Read the model definition and answer for the solid it produces. Units are mm, in the model's axes. Face numbers are marked on the shaded views. A direction names the side the tool comes from. Give positions to 0.01 mm unless a question says otherwise; leave off trailing zeros. Loops run counter-clockwise (first coordinate to the right, second up) from the corner with the lowest first, then second, coordinate; pieces in that order, holes last. Notation, with made-up numbers: (66, 65.5) - (112, 65.5) arc R15 ccw to (112, 84.5) - close; hole circle Ø2 at (56.25, 1.5). An arc over 180 degrees is marked (long way). Use a Markdown table: item, result. Add a question column.
Item 1: For a pull along Y with two mould halves and no side action, classify the marked faces 3, 4, 5 and 6 as +Y half, -Y half, draft (parallel to the pull), parting line (faces both ways), or undercut.
Item 2: Consider probe 1 along X at (y, z) = (19.5, 25.5); probe 2 along Y at (x, z) = (5.5, 19.75); probe 3 along X at (y, z) = (10, 24). Determine where each line is inside the solid, lowest interval first. Write a range as [from, to].
Item 3: A cutting plane is placed at C-C (x = -20). Determine the outline of the cut face in (y, z), plus the area to 3 significant figures.
Item 4: Which of the six approach directions +Z, -Z, +X, -X, +Y, -Y give full straight-line access (tool end or side, diameter ignored) to the marked faces 1 and 2?
Item 5: A cutting plane is placed at B-B (z = 25). Determine the outline of the cut face in (x, y).
Item 6: A cutting plane is placed at D-D (z = 19.75). Determine the outline of the cut face in (x, y).
Item 7: Each of these flat-tipped pins is pushed along its axis until it touches: P1, Ø5, axis at x = -20.44, y = 30.84, coming from the +Z side; P2, Ø1.5, axis at x = 10, y = 22, coming from the -Z side; P3, Ø1.5, axis at x = 4.5, y = 21.5, coming from the -Z side; P4, Ø3, axis at x = 19.56, y = 10.84, coming from the -Z side. Where does it stop, or does it pass through?
Item 8: A cutting plane is placed at A-A (x = 14.5). Determine the outline of the cut face in (y, z).
from build123d import *

# Parameters (mm, degrees)
SKETCH1_W           = 50
SKETCH1_H           = 10
BOSS_EXTRUDE1_DEPTH = 40
CUT_EXTRUDE1_REACH  = 12
SKETCH2_R           = 1.75
SKETCH3_R           = 3
CUT_EXTRUDE2_DEPTH  = 4
SKETCH5_R           = 2.5
CUT_EXTRUDE3_DEPTH  = 8
SKETCH6_W           = 20
SKETCH6_H           = 5
CUT_EXTRUDE4_DEPTH  = 3


with BuildPart() as part:
    # Sketch1 → Boss-Extrude1 (new body)
    with BuildSketch(Plane(origin=(0, 0.83575208, 0), x_dir=(-1, 0, 0), z_dir=(0, 1, 0))):
        with Locations((0.444640388, 23.28984466)):
            Rectangle(SKETCH1_W, SKETCH1_H)
    extrude(amount=BOSS_EXTRUDE1_DEPTH)

    # Sketch2 → Cut-Extrude1 (cut, up to next)
    with BuildSketch(Plane.XY.offset(28.28984466), mode=Mode.PRIVATE) as cut_extrude1_sk1:
        with Locations((-20.444640388, 30.83575208)):
            Circle(SKETCH2_R)
    cut_extrude1_tool1 = extrude(cut_extrude1_sk1.sketch, amount=-CUT_EXTRUDE1_REACH, mode=Mode.PRIVATE) & part.part
    add(cut_extrude1_tool1.solids().sort_by_distance((-20.44464, 30.835752, 28.289845))[0], mode=Mode.SUBTRACT)
    # Sketch2 → Cut-Extrude1 (cut, up to next)
    with BuildSketch(Plane.XY.offset(28.28984466), mode=Mode.PRIVATE) as cut_extrude1_sk2:
        with Locations((-20.444640388, 10.83575208)):
            Circle(SKETCH2_R)
    cut_extrude1_tool2 = extrude(cut_extrude1_sk2.sketch, amount=-CUT_EXTRUDE1_REACH, mode=Mode.PRIVATE) & part.part
    add(cut_extrude1_tool2.solids().sort_by_distance((-20.44464, 10.835752, 28.289845))[0], mode=Mode.SUBTRACT)
    # Sketch2 → Cut-Extrude1 (cut, up to next)
    with BuildSketch(Plane.XY.offset(28.28984466), mode=Mode.PRIVATE) as cut_extrude1_sk3:
        with Locations((19.555359612, 10.83575208)):
            Circle(SKETCH2_R)
    cut_extrude1_tool3 = extrude(cut_extrude1_sk3.sketch, amount=-CUT_EXTRUDE1_REACH, mode=Mode.PRIVATE) & part.part
    add(cut_extrude1_tool3.solids().sort_by_distance((19.55536, 10.835752, 28.289845))[0], mode=Mode.SUBTRACT)
    # Sketch2 → Cut-Extrude1 (cut, up to next)
    with BuildSketch(Plane.XY.offset(28.28984466), mode=Mode.PRIVATE) as cut_extrude1_sk4:
        with Locations((19.555359612, 30.83575208)):
            Circle(SKETCH2_R)
    cut_extrude1_tool4 = extrude(cut_extrude1_sk4.sketch, amount=-CUT_EXTRUDE1_REACH, mode=Mode.PRIVATE) & part.part
    add(cut_extrude1_tool4.solids().sort_by_distance((19.55536, 30.835752, 28.289845))[0], mode=Mode.SUBTRACT)

    # Sketch3 → Cut-Extrude2 (cut)
    with BuildSketch(Plane.XY.offset(28.28984466)):
        with Locations((-20.444640388, 30.83575208)):
            Circle(SKETCH3_R)
        with Locations((-20.444640388, 10.83575208)):
            Circle(SKETCH3_R)
        with Locations((19.555359612, 10.83575208)):
            Circle(SKETCH3_R)
        with Locations((19.555359612, 30.83575208)):
            Circle(SKETCH3_R)
    extrude(amount=-CUT_EXTRUDE2_DEPTH, mode=Mode.SUBTRACT)

    # Sketch5 → Cut-Extrude3 (cut)
    with BuildSketch(Plane(origin=(0, 0, 18.28984466), x_dir=(-1, 0, 0), z_dir=(0, 0, -1))):
        with Locations((5.444640388, 20.83575208)):
            Circle(SKETCH5_R)
        with Locations((-4.555359612, 20.83575208)):
            Circle(SKETCH5_R)
    extrude(amount=-CUT_EXTRUDE3_DEPTH, mode=Mode.SUBTRACT)

    # Sketch6 → Cut-Extrude4 (cut)
    with BuildSketch(Plane(origin=(0, 0, 18.28984466), x_dir=(-1, 0, 0), z_dir=(0, 0, -1))):
        with Locations((15.444640388, 20.83575208)):
            Rectangle(SKETCH6_W, SKETCH6_H)
        with Locations((-14.555359612, 20.83575208)):
            Rectangle(SKETCH6_W, SKETCH6_H)
    extrude(amount=-CUT_EXTRUDE4_DEPTH, mode=Mode.SUBTRACT)


solid = part.part
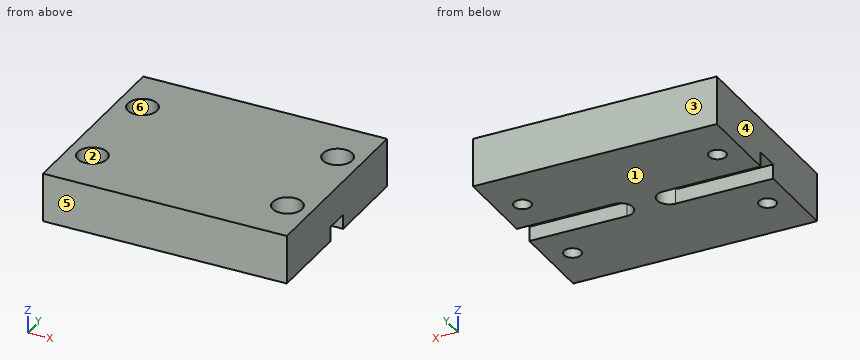
Geometry says:
| question | item | result |
|---|---|---|
| 1 | face 3 | +Y half |
| 1 | face 4 | draft |
| 1 | face 5 | -Y half |
| 1 | face 6 | undercut |
| 2 | probe 1 | [-25.44, -7.56], [-3.33, 2.44], [6.67, 24.56] |
| 2 | probe 2 | [0.84, 18.34], [23.34, 40.84] |
| 2 | probe 3 | [-25.44, -21.98], [-18.91, 18.02], [21.09, 24.56] |
| 3 | outline | (0.84, 18.29) - (9.14, 18.29) - (9.14, 24.29) - (7.87, 24.29) - (7.87, 28.29) - (0.84, 28.29) - close; (12.53, 18.29) - (18.34, 18.29) - (18.34, 21.29) - (23.34, 21.29) - (23.34, 18.29) - (29.14, 18.29) - (29.14, 24.29) - (27.87, 24.29) - (27.87, 28.29) - (13.8, 28.29) - (13.8, 24.29) - (12.53, 24.29) - close; (32.53, 18.29) - (40.84, 18.29) - (40.84, 28.29) - (33.8, 28.29) - (33.8, 24.29) - (32.53, 24.29) - close |
| 3 | area | 297 mm² |
| 4 | face 1 | -Z, +X, -X, +Y, -Y |
| 4 | face 2 | +Z |
| 5 | outline | (-25.44, 0.84) - (24.56, 0.84) - (24.56, 40.84) - (-25.44, 40.84) - close; hole circle Ø6 at (-20.44, 10.84); hole circle Ø6 at (-20.44, 30.84); hole circle Ø5 at (-5.44, 20.84); hole circle Ø5 at (4.56, 20.84); hole circle Ø6 at (19.56, 10.84); hole circle Ø6 at (19.56, 30.84) |
| 6 | outline | (-25.44, 0.84) - (24.56, 0.84) - (24.56, 18.34) - (4.56, 18.34) arc R2.5 cw to (4.56, 23.34) - (24.56, 23.34) - (24.56, 40.84) - (-25.44, 40.84) - (-25.44, 23.34) - (-5.44, 23.34) arc R2.5 cw to (-5.44, 18.34) - (-25.44, 18.34) - close; hole circle Ø3.5 at (-20.44, 10.84); hole circle Ø3.5 at (-20.44, 30.84); hole circle Ø3.5 at (19.56, 10.84); hole circle Ø3.5 at (19.56, 30.84) |
| 7 | P1 | z = 24.29 |
| 7 | P2 | z = 21.29 |
| 7 | P3 | z = 26.29 |
| 7 | P4 | through |
| 8 | outline | (0.84, 18.29) - (18.34, 18.29) - (18.34, 21.29) - (23.34, 21.29) - (23.34, 18.29) - (40.84, 18.29) - (40.84, 28.29) - (0.84, 28.29) - close |
